Here's the drawing with two shaded views (mm, measured from the low corner). I have some questions. A direction names the side the tool comes from. Coordinates: 2 decimals unless noted, no trailing zeros. Loops run counter-clockwise (first coordinate to the right, second up) from the corner with the lowest first, then second, coordinate; pieces in that order, holes last.
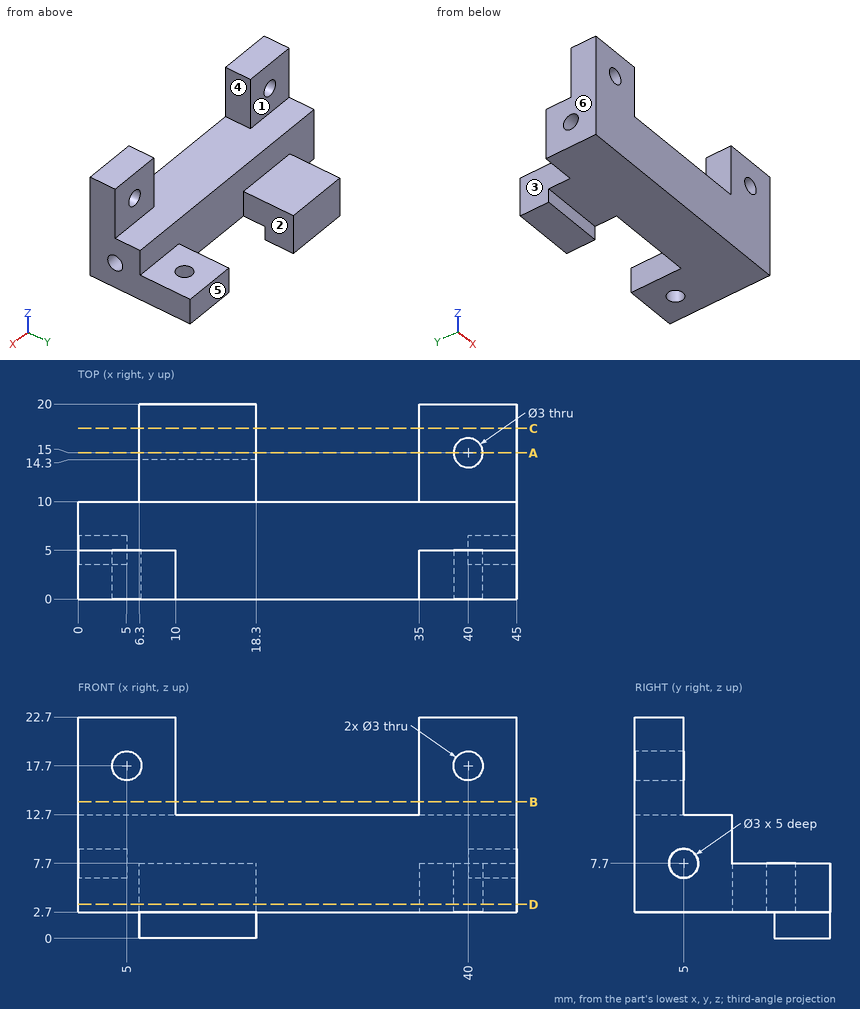
(1) I want a section at B-B on z = 14. Write out the boundary of the cut face in (x, y).
Check values:
outline: (0, 0) - (10, 0) - (10, 5) - (0, 5) - close; (35, 0) - (45, 0) - (45, 5) - (35, 5) - close
(2) I want a section at A-A on y = 15. Write out the boundary of the cut face in (x, z).
Check values:
outline: (6.3, 0) - (18.3, 0) - (18.3, 7.7) - (6.3, 7.7) - close; (35, 2.7) - (38.5, 2.7) - (38.5, 7.7) - (35, 7.7) - close; (41.5, 2.7) - (45, 2.7) - (45, 7.7) - (41.5, 7.7) - close
(3) I want a section at C-C on y = 17.5. Write out the boundary of the cut face in (x, z).
Check values:
outline: (6.3, 0) - (18.3, 0) - (18.3, 7.7) - (6.3, 7.7) - close; (35, 2.7) - (45, 2.7) - (45, 7.7) - (35, 7.7) - close
(4) If we mould it in two halves opening along X, with no side actions, what happens to the marked faces 4, 5 and 6? For each: released by +X, released by -X, zero draft, split by the parting line, or undercut.
Check values:
face 4: undercut
face 5: zero draft
face 6: released by -X
(5) If I drill on probe 1 along Y at (x, z) = (2.05, 7.7); probe 2 along Y at (x, z) = (40, 5.8); probe 3 along Z at (x, y) = (21.5, 4.75), over which ranges is the centre line in solid material (lowest first)?
Check values:
probe 1: y = 0 to 3.5, 6.5 to 10
probe 2: y = 0 to 13.5, 16.5 to 20
probe 3: z = 2.7 to 12.7
(6) I want a section at D-D on z = 3.5. Write out the boundary of the cut face in (x, y).
Check values:
outline: (0, 0) - (45, 0) - (45, 20) - (35, 20) - (35, 10) - (18.3, 10) - (18.3, 20) - (6.3, 20) - (6.3, 10) - (0, 10) - close; hole circle Ø3 at (40, 15)
(7) Which directions (+Z, -Z, +X, -X, +Y, -Y) give clear straight access to the entire face, cutting with the end or side of a thin tool? Please do the marked faces 1, 2 and 3.
Check values:
face 1: +Z, +X, -X, +Y
face 2: +Z, -Z, +Y
face 3: +Z, -Z, -X, +Y
(8) I'm going to push flat-ended pins straight in: pin 1 (1.5 mm diameter, centred on y = 5.5, z = 8, fed in from -X); pin 2 (4 mm diameter, centred on y = 15.5, z = 5.5, fed in from -X); pin 3 (3 mm diameter, centred on x = 38, y = 17.5, fed in from +Z). Where does each tip first touch, or does it pass through?
Check values:
pin 1: stops at x = 5
pin 2: stops at x = 6.3
pin 3: stops at z = 7.7
